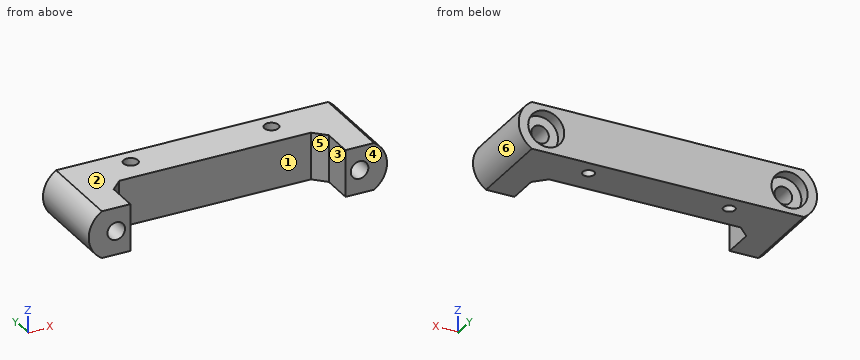
from build123d import *

# Parameters (mm, degrees)
SKETCH1_R               = 1
BOSS_EXTRUDE1_DEPTH     = 8
SKETCH2_R               = 1.5
CUT_EXTRUDE1_DEPTH      = 15.75
BOSS_EXTRUDE2_DEPTH     = 14.75
SKETCH5_R               = 3.075
CUT_EXTRUDE2_DEPTH      = 1
CUT_EXTRUDE2_DEPTH_BACK = 2
CHAMFER2_SIZE           = 2
SKETCH6_R               = 1.225
CUT_EXTRUDE3_DEPTH      = 5


with BuildPart() as part:
    # Sketch1 → Boss-Extrude1 (new body)
    with BuildSketch(Plane.XY):
        Polygon((18.35, 7.35), (18.35, 0), (23.2, 0), (23.2, 14.75), (-23.2, 14.75), (-23.2, 0), (-18.35, 0), (-18.35, 7.35), align=None)
        with Locations((-12, 11.85)):
            Circle(SKETCH1_R, mode=Mode.SUBTRACT)
        with Locations((12, 11.85)):
            Circle(SKETCH1_R, mode=Mode.SUBTRACT)
    extrude(amount=BOSS_EXTRUDE1_DEPTH)

    # Sketch2 → Cut-Extrude1 (cut, through all)
    with BuildSketch(Plane.XZ):
        with Locations((-20.75, 4)):
            Circle(SKETCH2_R)
        with Locations((20.75, 4)):
            Circle(SKETCH2_R)
    extrude(amount=-CUT_EXTRUDE1_DEPTH, mode=Mode.SUBTRACT)

    # Sketch3 → Boss-Extrude2 (add)
    with BuildSketch(Plane(origin=(0, 14.75, 0), x_dir=(1, 0, 0), z_dir=(0, 1, 0))):
        with BuildLine():
            Line((23.2, -8), (23.2, 0))
            ThreePointArc((23.2, 0), (25.440682253, -4), (23.2, -8))
        make_face()
        with BuildLine():
            Line((-23.2, -8), (-23.2, 0))
            ThreePointArc((-23.2, 0), (-25.440682253, -4), (-23.2, -8))
        make_face()
    extrude(amount=-BOSS_EXTRUDE2_DEPTH)

    # Sketch5 → Cut-Extrude2 (cut, two sides)
    with BuildSketch(Plane(origin=(0, 14.75, 0), x_dir=(1, 0, 0), z_dir=(0, 1, 0))) as cut_extrude2_sk:
        with Locations((20.75, -4)):
            Circle(SKETCH5_R)
        with Locations((-20.75, -4)):
            Circle(SKETCH5_R)
    extrude(amount=CUT_EXTRUDE2_DEPTH, mode=Mode.SUBTRACT)
    extrude(cut_extrude2_sk.sketch, amount=-CUT_EXTRUDE2_DEPTH_BACK, mode=Mode.SUBTRACT)

    # Chamfer2
    chamfer2_edges = [part.edges().sort_by_distance(p)[0] for p in [
        (-18.35, 7.35, 4),
        (18.35, 7.35, 4),
    ]]
    chamfer(chamfer2_edges, length=CHAMFER2_SIZE)

    # Sketch6 → Cut-Extrude3 (cut)
    with BuildSketch(Plane.XY.offset(8)):
        with Locations((-12, 11.85)):
            Circle(SKETCH6_R)
        with Locations((12, 11.85)):
            Circle(SKETCH6_R)
    extrude(amount=-CUT_EXTRUDE3_DEPTH, mode=Mode.SUBTRACT)


solid = part.part
Work out the finished part from the listing and answer in its coordinate system (mm). Face numbers are marked on the shaded views. A direction names the side the tool comes from. Round coordinates to 2 decimals unless told otherwise and drop trailing zeros. Write each loop counter-clockwise with the first axis right and the second up, starting at its lowest first coordinate (ties: lowest second). Pieces come first, ordered by that corner, then holes. Notation, with made-up numbers: M 7,-21 L 61,-21 A20 ccw 61,15 Z; hole C 81.5,-14.5 d8. An arc over 180 degrees is marked long. Use a Markdown table: item, result.
1) The part is cut by section C-C on y = 2.5. Give the vertices of the cut face in (x, z).
Taken from the geometry:
| item | result |
|---|---|
| outline | M -23.2,0 L -18.35,0 L -18.35,8 L -23.2,8 A4.69 ccw Z; M 18.35,0 L 23.2,0 A4.69 ccw 23.2,8 L 18.35,8 Z; hole C -20.75,4 d3; hole C 20.75,4 d3 |
2) Determine the mould class of the marked faces 3, 4, 5 and 6 for opening direction X: pulls with the +X half, pulls with the -X half, needs draft (parallel to the pull), parting line crosses it, or undercut.
Taken from the geometry:
| item | result |
|---|---|
| face 3 | undercut |
| face 4 | needs draft |
| face 5 | undercut |
| face 6 | pulls with the +X half |
3) Which of the six approach directions +Z, -Z, +X, -X, +Y, -Y give full straight-line access (tool end or side, diameter ignored) to the marked faces 1 and 2?
Taken from the geometry:
| item | result |
|---|---|
| face 1 | +Z, -Z, -Y |
| face 2 | +Z, +X, -X, +Y, -Y |
4) Flat-ended cylindrical pins translate along their axes: pin 1 (4 mm diameter, centred on x = -20.75, z = 4, fed in from +Y); pin 2 (1.5 mm diameter, centred on x = 9.5, z = 1.5, fed in from -Y). Find the tip coordinate at first contact, or state that the pin passes through.
Taken from the geometry:
| item | result |
|---|---|
| pin 1 | stops at y = 12.75 |
| pin 2 | stops at y = 7.35 |
5) The part is cut by section D-D on x = -20.75. Give the vertices of the cut face in (y, z) (3 decimals).
Taken from the geometry:
| item | result |
|---|---|
| outline | M 0,0 L 14.75,0 L 14.75,0.925 L 12.75,0.925 L 12.75,2.5 L 0,2.5 Z; M 0,5.5 L 12.75,5.5 L 12.75,7.075 L 14.75,7.075 L 14.75,8 L 0,8 Z |
6) Consider line 1 (Z direction, x = 21, y = 13.75); line 2 (X direction, y = 11.85, z = 0.7); line 3 (Y direction, x = 12, z = 3.25) (3 decimals). Determine where each line is inside the solid, lowest interval first. Write a range as [from, to].
Taken from the geometry:
| item | result |
|---|---|
| line 1 | z = [0, 0.94], [7.06, 8] |
| line 2 | x = [-24.08, -13], [-11, 11], [13, 24.08] |
| line 3 | y = [7.35, 10.625], [13.075, 14.75] |
7) The part is cut by section A-A on z = 4. Give the vertices of the cut face in (x, y) (3 decimals), plus the area to 3 significant figures.
Taken from the geometry:
| item | result |
|---|---|
| outline | M -25.441,0 L -22.25,0 L -22.25,12.75 L -23.825,12.75 L -23.825,14.75 L -25.441,14.75 Z; M -19.25,0 L -18.35,0 L -18.35,5.35 L -16.35,7.35 L 16.35,7.35 L 18.35,5.35 L 18.35,0 L 19.25,0 L 19.25,12.75 L 17.675,12.75 L 17.675,14.75 L -17.675,14.75 L -17.675,12.75 L -19.25,12.75 Z; M 22.25,0 L 25.441,0 L 25.441,14.75 L 23.825,14.75 L 23.825,12.75 L 22.25,12.75 Z; hole C -12,11.85 d2.45; hole C 12,11.85 d2.45 |
| area | 374 mm2 |
8) The part is cut by section B-B on y = 11.85. Give the vertices of the cut face in (x, z) (3 decimals), plus the area to 3 significant figures.
Taken from the geometry:
| item | result |
|---|---|
| outline | M -23.2,0 L -13,0 L -13,3 L -13.225,3 L -13.225,8 L -23.2,8 A4.691 ccw Z; M -11,0 L 11,0 L 11,3 L 10.775,3 L 10.775,8 L -10.775,8 L -10.775,3 L -11,3 Z; M 13,0 L 23.2,0 A4.691 ccw 23.2,8 L 13.225,8 L 13.225,3 L 13,3 Z; hole C -20.75,4 d3; hole C 20.75,4 d3 |
| area | 346 mm2 |
